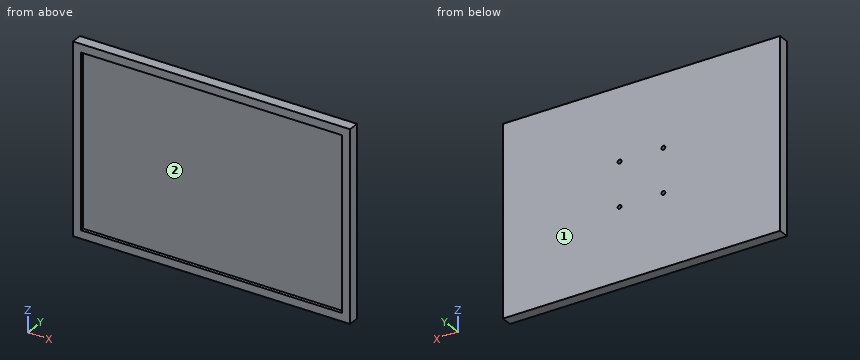
```python
from build123d import *

# Parameters (mm, degrees)
F0_W     = 642.62
F0_H     = 437.896
F1_DEPTH = 25.4
F3_D     = 8.89
F3_DEPTH = 8.89
F3_TIP   = 2.6708254516
F4_W     = 604.52
F4_H     = 399.796
F5_DEPTH = 7.62


with BuildPart() as f1:
    # F0 (on Front) → F1 (new body)
    with BuildSketch(Plane.XZ):
        with Locations((321.31, 218.948)):
            Rectangle(F0_W, F0_H)
    extrude(amount=F1_DEPTH)

    # F3
    with Locations(Plane(origin=(0, 0, 0), x_dir=(-1, 0, 0), z_dir=(0, 1, 0))):
        with Locations((-372.11, 269.748), (-270.51, 269.748), (-270.51, 168.148), (-372.11, 168.148)):
            Hole(F3_D / 2, depth=F3_DEPTH)
            with Locations((0, 0, -(F3_DEPTH + F3_TIP / 2))):  # 118° drill point
                Cone(0, F3_D / 2, F3_TIP, mode=Mode.SUBTRACT)

    # F4 (on face) → F5 (cut)
    with BuildSketch(Plane.XZ.offset(25.4)):
        with Locations((321.31, 218.948)):
            Rectangle(F4_W, F4_H)
    extrude(amount=-F5_DEPTH, mode=Mode.SUBTRACT)


solid = f1.part
```
Input: part model. Units: mm. Frame: model coordinates. Face numbers are marked on the shaded views. Give positions to 0.01 mm unless a question says otherwise; leave off trailing zeros. Loops run counter-clockwise (first coordinate to the right, second up) from the corner with the lowest first, then second, coordinate; pieces in that order, holes last. Notation, with made-up numbers: M 20.25,86 L 44.25,86 A6 cw 44.25,97 Z; hole C 34,77.25 d10. An arc over 180 degrees is marked long. Answer as CSV lines item,"result". Start each with the question number.
1. Pull-direction query (Z, two-part tool) for the marked faces 1 and 2; classes: released by +Z, released by -Z, zero draft, split by the parting line, or undercut.
2. Section B-B on z = 71.5. Return loops of the section in (x, y).
3. Section A-A on x = 343.5. Return loops of the section in (y, z), plus the area to 3 significant figures.
4. Pin query (flat end, axial travel): P1, Ø10, axis at x = 120.5, z = 101.5, coming from the -Y side; P2, Ø5.5, axis at x = 270.51, z = 168.148, coming from the +Y side; P3, Ø8, axis at x = 372.11, z = 168.148, coming from the +Y side. Return the tip coordinate at first contact, or that it passes through.
5. Line query: L1, parallel to Z at x = 372.11, y = -2.5; L2, parallel to Z at x = 490.5, y = -18; L3, parallel to X at y = -3.75, z = 269. Output: solid intervals per line, ascending.
Computed values:
1,face 1,"zero draft"
1,face 2,"undercut"
2,outline,"M 0,-25.4 L 19.05,-25.4 L 19.05,-17.78 L 623.57,-17.78 L 623.57,-25.4 L 642.62,-25.4 L 642.62,0 L 0,0 Z"
3,outline,"M -25.4,0 L 0,0 L 0,437.9 L -25.4,437.9 L -25.4,418.85 L -17.78,418.85 L -17.78,19.05 L -25.4,19.05 Z"
3,area,"8,080 mm²"
4,P1,"stops at y = -17.78"
4,P2,"stops at y = -9.91"
4,P3,"stops at y = -9.16"
5,L1,"z = 0 to 163.7, 172.59 to 265.3, 274.19 to 437.9"
5,L2,"z = 0 to 19.05, 418.85 to 437.9"
5,L3,"x = 0 to 266.13, 274.89 to 367.73, 376.49 to 642.62"
